For this review, take the finished solid that the model builds, in its own axes (mm). Coordinates: 2 decimals unless noted, no trailing zeros. Write each loop counter-clockwise with the first axis right and the second up, starting at its lowest first coordinate (ties: lowest second). Pieces come first, ordered by that corner, then holes. Notation, with made-up numbers: (53, 27.5) -> (67, 27.5) arc R25 cw to (67, 62.5) -> close; hole circle Ø7 at (52.5, 3.25). An arc over 180 degrees is marked (long way). One line per item, written item: value. Start each with the question number.
1) Add section D-D (z = -32). State the section outline as (x, y) points.
2) Mouldability with a two-part tool opening along Z and no side actions: class faces 1 (the flat face through (1.48, 9.8, -20.85)), 2 (the cylindrical face through (1.479, -3.022, -41.591)), 3 (the flat face through (0, 0, -9)) as released by +Z, released by -Z, zero draft, split by the parting line, or undercut.
3) Add section A-A (z = -40.5). State the section outline as (x, y) points, and give its area (3 significant figures).
4) For probe 1 along Z at (x, y) = (2.8, 3.5); probe 2 along Y at (x, z) = (2.15, -21); probe 3 along Z at (x, y) = (1.7, -14.5), list the stretches that pass through material, from the lowest coordinate up. Write a range as from..to.
5) Add section B-B (y = -3.5). State the section outline as (x, z) points.
6) Add section C-C (x = 1.9). State the section outline as (y, z) points, and give its area (3 significant figures).
Autodesk Inventor part; units mm, degrees
ref_plane "YZ Plane" through (0, 0, 0) normal (1, 0, 0) x (0, 1, 0)
ref_plane "XZ Plane" through (0, 0, 0) normal (0, 1, 0) x (-1, 0, 0)
ref_plane "XY Plane" through (0, 0, 0) normal (0, 0, 1) x (1, 0, 0)
sketch "Эскиз1" plane through (0, 0, 0) normal (1, 0, 0) x (0, 1, 0)
  circle A0 centre (35.2311, -22.6062) radius 9.3
  circle A1 centre (0, -38.8201) radius 6.1 construction
  circle A2 centre (0, 0) radius 4.85 construction
  circle A3 centre (35.8147, -49.5529) radius 3.55
  line L0 (6.0968, -38.6237) -> (4.8475, 0.1562) construction
  line L1 (-4.8475, 0.1562) -> (-6.0968, -38.6237) construction
  line L2 (0, 0) -> (0, -38.8201) construction
  circle A4 centre (0, -38.8201) radius 4.1
  circle A5 centre (0, 0) radius 2.25
  circle A6 centre (0, -38.8201) radius 15 construction
  circle A7 centre (0, 0) radius 14 construction
  circle A8 centre (0, -38.8201) radius 7.6
  circle A9 centre (0, 0) radius 7 construction
  line L3 (7.5465, -39.7207) -> (12.114, -1.4456)
  line L4 (-7.5465, -39.7207) -> (-12.114, -1.4456)
  circle A10 centre (0, 0) radius 8.8 construction
  circle A11 centre (0, 0) radius 12.2
  circle A12 centre (6.8983, -19.8347) radius 1.6
  circle A13 centre (-7.3019, -16.4524) radius 1.6
  point P0 (-7, 0)
  point P1 (-7.5465, -39.7207)
  point P2 (-12.114, -1.4456)
  dimension "d0" = 18.6
  dimension "d1" = 12.2
  dimension "d2" = 9.7
  dimension "d3" = 7.1
  dimension "d8" = 38.8201
  dimension "d13" = 38.8
  dimension "d14" = 38.8
  dimension "d23" = 8.2
  dimension "d24" = 4.5
  dimension "d25" = 30
  dimension "d26" = 28
  dimension "d28" = 14
  dimension "d31" = 17.6
  dimension "d32" = 3.4
  dimension "d56" = 3.5
  dimension "d58" = 3.2
  dimension "d59" = 3
  dimension "d60" = 21
  dimension "d61" = 3.2
  dimension "d62" = 3
  dimension "d63" = 18
extrude "Выдавливание4" add sketch "Эскиз1" along normal blind 3 contours A5 | A8 | A8 L4 A11 L3 | A11
sketch "Эскиз4" plane through (0, 0, 0) normal (-1, 0, 0) x (0, 0, 1)
  circle A0 centre (-6.2, 6.2) radius 1.4
  circle A1 centre (-38.8201, 0) radius 4.1 construction
  arc A2 (-1.4456, -12.114) -> (-1.4456, 12.114) centre (0, 0) ccw construction
  line L0 (-39.7207, 7.5465) -> (-1.4456, 12.114) construction
  arc A3 (-39.7207, 7.5465) -> (-39.7207, -7.5465) centre (-38.8201, 0) ccw construction
  line L1 (-1.4456, -12.114) -> (-39.7207, -7.5465) construction
  line L2 (0, 0) -> (0, 12.2) construction
  arc A4 (-1.4456, -12.114) -> (-1.4456, 12.114) centre (0, 0) ccw construction
  line L3 (0, 0) -> (12.2, 0) construction
  circle A5 centre (6.2, 6.2) radius 1.4
  circle A6 centre (-6.2, -6.2) radius 1.4
  circle A7 centre (6.2, -6.2) radius 1.4
  dimension "d33" = 2.8
  dimension "d34" = 12.4
  dimension "d35" = 12.4
extrude "Выдавливание5" [suppressed]
sketch "Эскиз5" plane through (3, 0, 0) normal (1, 0, 0) x (0, 0, -1)
  circle A0 centre (0, 0) radius 3.75
  dimension "d38" = 7.5
extrude "Выдавливание6" [suppressed]
sketch "Эскиз6" plane through (3, 0, 0) normal (1, 0, 0) x (0, 0, -1)
  circle A0 centre (0, -18) radius 2
  circle A1 centre (38.8201, 0) radius 4.1 construction
  line L0 (39.7207, 7.5465) -> (1.4456, 12.114) construction
  arc A2 (1.4456, 12.114) -> (1.4456, -12.114) centre (0, 0) ccw construction
  line L1 (1.4456, -12.114) -> (39.7207, -7.5465) construction
  arc A3 (39.7207, -7.5465) -> (39.7207, 7.5465) centre (38.8201, 0) ccw construction
  line L2 (0, 0) -> (0, -26.6004) construction
  circle A4 centre (0, 0) radius 14 construction
  line L3 (-10.8605, -5.5578) -> (-3.5608, -19.8222)
  arc A5 (0, -14) -> (-3.5608, -19.8222) centre (0, -18) ccw construction
  line L4 (2.8284, -20.8284) -> (12.911, -10.7458)
  line L5 (1.4456, -12.114) -> (39.7207, -7.5465) construction
  arc A6 (2.8284, -20.8284) -> (0, -14) centre (0, -18) ccw construction
  arc A7 (-3.5608, -19.8222) -> (2.8284, -20.8284) centre (0, -18) ccw
  line L6 (-10.8605, -5.5578) -> (-10.1465, -5.5578)
  line L7 (-10.1465, -5.5578) -> (-6.8136, -9.4237)
  line L8 (-6.8136, -9.4237) -> (5.1237, -10.512)
  line L9 (5.1237, -10.512) -> (12.911, -10.7458)
  dimension "d42" = 28
  dimension "d41" = 4
  dimension "d43" = 18
  dimension "d44" = 8
  dimension "d45" = 45
extrude "Выдавливание7" [suppressed]
sketch "Эскиз7" plane through (3, 0, 0) normal (1, 0, 0) x (0, 0, -1)
  line L0 (0, 0) -> (0, -29.4139) construction
  circle A0 centre (-9, -15.5885) radius 1.6
  line L1 (-9, -15.5885) -> (0, 0) construction
  circle A1 centre (0, 0) radius 14 construction
  circle A2 centre (0, 0) radius 18 construction
  arc A3 (-6.7, -19.5722) -> (-13.5823, -15.1855) centre (-9, -15.5885) ccw construction
  circle A4 centre (38.8201, 0) radius 4.1 construction
  line L2 (39.7207, 7.5465) -> (1.4456, 12.114) construction
  arc A5 (1.4456, 12.114) -> (1.4456, -12.114) centre (0, 0) ccw
  line L3 (1.4456, -12.114) -> (39.7207, -7.5465)
  arc A6 (39.7207, -7.5465) -> (39.7207, 7.5465) centre (38.8201, 0) ccw construction
  line L4 (-12.1531, 1.0686) -> (-13.5823, -15.1855)
  line L5 (-6.7, -19.5722) -> (7.4613, -11.3962)
  line L6 (1.4456, -12.114) -> (39.7207, -7.5465) construction
  arc A7 (-13.5823, -15.1855) -> (-6.7, -19.5722) centre (-9, -15.5885) ccw
  point P0 (7.4613, -11.3962)
  dimension "d48" = 3.2
  dimension "d49" = 330
  dimension "d50" = 28
  dimension "d51" = 4
  dimension "d53" = 30
  dimension "d57" = 3
extrude "Выдавливание8" add sketch "Эскиз7" against normal up to surface (3 mm away)
properties part number "left_wall_v1"
Numbers:
1. outline: (0, -8.47) -> (3, -8.47) -> (3, 8.47) -> (0, 8.47) -> close
2. face 1: released by -Z
2. face 2: undercut
2. face 3: zero draft
3. outline: (0, -7.41) -> (3, -7.41) -> (3, -3.74) -> (0, -3.74) -> close; (0, 3.74) -> (3, 3.74) -> (3, 7.41) -> (0, 7.41) -> close
3. area: 22.0 mm²
4. probe 1: -45.57..-40.96, -36.68..11.69
4. probe 2: -9.78..5.8, 7.99..9.78
4. probe 3: -2.09..7.83, 10.17..13.52
5. outline: (0, -45.57) -> (3, -45.57) -> (3, -40.96) -> (0, -40.96) -> close; (0, -36.68) -> (3, -36.68) -> (3, 12.55) -> (0, 12.55) -> close
6. outline: (-19.57, 6.7) -> (-11.4, -7.46) -> (-7.55, -39.72) arc R7.6 ccw to (7.55, -39.72) -> (12.11, -1.45) arc R12.2 ccw to (1.07, 12.15) -> (-15.19, 13.58) arc R4.6 ccw to start; hole circle Ø3.2 at (-15.59, 9); hole circle Ø3.2 at (-7.3, -16.45); hole circle Ø8.2 at (0, -38.82); hole circle Ø3.2 at (6.9, -19.83)
6. area: 1,160 mm²
